The listing builds one solid part. Answer for the finished solid, in the listing's coordinates (mm). A direction names the side the tool comes from. Round coordinates to 2 decimals unless told otherwise and drop trailing zeros. Write each loop counter-clockwise with the first axis right and the second up, starting at its lowest first coordinate (ties: lowest second). Pieces come first, ordered by that corner, then holes.
(1) Each of these flat-tipped pins is pushed along its axis until it touches: pin 1 Ø6 at (x, z) = (-21.5, 214) entering from -Y; pin 2 Ø1.5 at (x, y) = (13.5, -21.5) entering from +Z; pin 3 Ø1 at (x, z) = (-1.5, 70) entering from +Y. Where does it stop, or does it pass through?
(2) A cutting plane is placed at A-A, the plane x = 0. Give the vertices of the cut face in (y, z) (3 decimals), and give its area (3 significant figures).
(3) Find the intervals of material crossed by probe 1 along Z at (x, y) = (18, -23); probe 2 along Z at (x, y) = (-3.5, -32); probe 3 along X at (y, z) = (12.5, 173), in increasing order.
(4) For faces 1 (the face through (7, -14, 302.26)), 2 (the face through (-6.9, 13.4, 8.89)), 3 (the face through (0, 0, 311.15)), determine the directions among +Z, -Z, +X, -X, +Y, -Y from which every point of the face is accessible in a straight line to the end or side of a thin tool.
(5) A cutting plane is placed at C-C, the plane z = 198. Give the vertices of the cut face in (x, y).
from build123d import *

# Parameters (mm, degrees)
SKETCH1_R           = 14.732
BOSS_EXTRUDE1_DEPTH = 8.89
SKETCH2_R           = 31.75
BOSS_EXTRUDE2_DEPTH = 270.51
SKETCH3_R           = 34.925
BOSS_EXTRUDE3_DEPTH = 22.86
FILLET1_R           = 2.54


with BuildPart() as part:
    # Sketch1 → Boss-Extrude1 (new body)
    with BuildSketch(Plane.XY):
        Circle(SKETCH1_R)
    boss_extrude1 = extrude(amount=BOSS_EXTRUDE1_DEPTH)

    # Sketch2 → Boss-Extrude2 (add)
    with BuildSketch(Plane.XY.offset(8.89)):
        Circle(SKETCH2_R)
    extrude(amount=BOSS_EXTRUDE2_DEPTH)

    # Sketch3 → Boss-Extrude3 (add)
    with BuildSketch(Plane.XY.offset(279.4)):
        Circle(SKETCH3_R)
    extrude(amount=BOSS_EXTRUDE3_DEPTH)

    # Mirror1: Boss-Extrude1 across plane
    add(boss_extrude1.mirror(Plane(origin=(0, 0, 155.575), x_dir=(1, 0, 0), z_dir=(0, 0, -1))))

    # Fillet1
    fillet1_edges = [part.edges().sort_by_distance(p)[0] for p in [
        (-14.732, 0, 311.15),
        (-14.732, 0, 0),
        (-31.75, 0, 8.89),
        (-34.925, 0, 279.4),
        (-34.925, 0, 302.26),
    ]]
    fillet(fillet1_edges, radius=FILLET1_R)


solid = part.part
Solutions:
1. pin 1: stops at y = -25.8
1. pin 2: stops at z = 302.26
1. pin 3: stops at y = 31.73
2. outline: (-34.925, 281.94) arc R2.54 ccw to (-32.385, 279.4) - (-31.75, 279.4) - (-31.75, 11.43) arc R2.54 ccw to (-29.21, 8.89) - (-14.732, 8.89) - (-14.732, 2.54) arc R2.54 ccw to (-12.192, 0) - (12.192, 0) arc R2.54 ccw to (14.732, 2.54) - (14.732, 8.89) - (29.21, 8.89) arc R2.54 ccw to (31.75, 11.43) - (31.75, 279.4) - (32.385, 279.4) arc R2.54 ccw to (34.925, 281.94) - (34.925, 299.72) arc R2.54 ccw to (32.385, 302.26) - (14.732, 302.26) - (14.732, 308.61) arc R2.54 ccw to (12.192, 311.15) - (-12.192, 311.15) arc R2.54 ccw to (-14.732, 308.61) - (-14.732, 302.26) - (-32.385, 302.26) arc R2.54 ccw to (-34.925, 299.72) - close
2. area: 19,300 mm2
3. probe 1: z = 8.89 to 302.26
3. probe 2: z = 279.4 to 302.26
3. probe 3: x = -29.19 to 29.19
4. face 1: +Z
4. face 2: -Z
4. face 3: +Z, +X, -X, +Y, -Y
5. outline: circle Ø63.5 at (0, 0)
